Read the model definition and answer for the solid it produces. Units are mm, in the model's axes. Round coordinates to 2 decimals unless told otherwise and drop trailing zeros. Order: outer loops, then holes, each group sorted by start corner. A loop starts at its lowest first (then second) coordinate and runs counter-clockwise, first axis right, second up.
from build123d import *

# Parameters (mm, degrees)
ESQUISSE1_W      = 20
ESQUISSE1_H      = 15
ESQUISSE1_R      = 4
EXTRUSION1_DEPTH = 16.5
ESQUISSE2_R      = 2
EXTRUSION3_DEPTH = 16


with BuildPart() as part:
    # Esquisse1 → Extrusion1 (new body)
    with BuildSketch(Plane.XY):
        with Locations((-10, -7.5)):
            Rectangle(ESQUISSE1_W, ESQUISSE1_H)
        with Locations((-10, -7.5)):
            Circle(ESQUISSE1_R, mode=Mode.SUBTRACT)
    extrude(amount=EXTRUSION1_DEPTH)

    # Esquisse2 → Extrusion3 (cut, through all)
    with BuildSketch(Plane(origin=(0, 0, 0), x_dir=(1, 0, 0), z_dir=(0, 1, 0))):
        with Locations((-17, -8.25)):
            Circle(ESQUISSE2_R)
        with Locations((-3, -8.25)):
            Circle(ESQUISSE2_R)
    extrude(amount=-EXTRUSION3_DEPTH, mode=Mode.SUBTRACT)


solid = part.part
Q1. A cutting plane is placed at B-B, the plane x = -17. Give the vertices of the cut face in (y, z), plus the area to 4 significant figures.
Outcome:
outline: (-15, 0) - (0, 0) - (0, 6.25) - (-15, 6.25) - close; (-15, 10.25) - (0, 10.25) - (0, 16.5) - (-15, 16.5) - close
area: 187.5 mm2
Q2. Straight lines are drawn through the part: probe 1 along Z at (x, y) = (-17, -5.5); probe 2 along X at (y, z) = (-8.75, 8.25); probe 3 along X at (y, z) = (-9.75, 8.5). For each, find the intervals that lie inside material, in ascending order.
Outcome:
probe 1: z = 0 to 6.25, 10.25 to 16.5
probe 2: x = -20 to -19, -15 to -13.8, -6.2 to -5, -1 to 0
probe 3: x = -20 to -18.98, -15.02 to -13.31, -6.69 to -4.98, -1.02 to 0
Q3. A cutting plane is placed at D-D, the plane z = 14.25. Give the vertices of the cut face in (x, y), plus the area to 3 significant figures.
Outcome:
outline: (-20, -15) - (0, -15) - (0, 0) - (-20, 0) - close; hole circle Ø8 at (-10, -7.5)
area: 250 mm2
Q4. For a pull along Z with two mould halves and no side action, classify faces 1 (the face through (-3.26, -7.395, 6.267)), 2 (the face through (-12.4, -4.1, 0)), 3 (the face through (-13.996, -7.324, 8.134)), 4 (the face through (-12.4, -4.1, 16.5)) as released by +Z, released by -Z, zero draft, split by the parting line, or undercut.
Outcome:
face 1: undercut
face 2: released by -Z
face 3: zero draft
face 4: released by +Z
Q5. A cutting plane is placed at A-A, the plane z = 8.25. Give the vertices of the cut face in (x, y), plus the area to 3 significant figures.
Outcome:
outline: (-20, -15) - (-19, -15) - (-19, 0) - (-20, 0) - close; (-15, -15) - (-5, -15) - (-5, 0) - (-15, 0) - close; (-1, -15) - (0, -15) - (0, 0) - (-1, 0) - close; hole circle Ø8 at (-10, -7.5)
area: 130 mm2
Q6. A cutting plane is placed at C-C, the plane y = -4. Give the vertices of the cut face in (x, z), plus the area to 3 significant figures.
Outcome:
outline: (-20, 0) - (-11.94, 0) - (-11.94, 16.5) - (-20, 16.5) - close; (-8.06, 0) - (0, 0) - (0, 16.5) - (-8.06, 16.5) - close; hole circle Ø4 at (-17, 8.25); hole circle Ø4 at (-3, 8.25)
area: 241 mm2
